The drawing under review shows one solid part. Ordinate dimensions are in mm from its lowest x, y, z. A direction names the side the tool comes from. Give positions to 0.01 mm unless a question says otherwise; leave off trailing zeros. Write each loop counter-clockwise with the first axis right and the second up, starting at its lowest first coordinate (ties: lowest second). Pieces come first, ordered by that corner, then holes. Notation, with made-up numbers: (30, -0.75) - (43, -0.75) arc R21 cw to (43, 32.25) - close; hole circle Ø9 at (32.5, 46). An arc over 180 degrees is marked (long way). Write item = value, one per line.
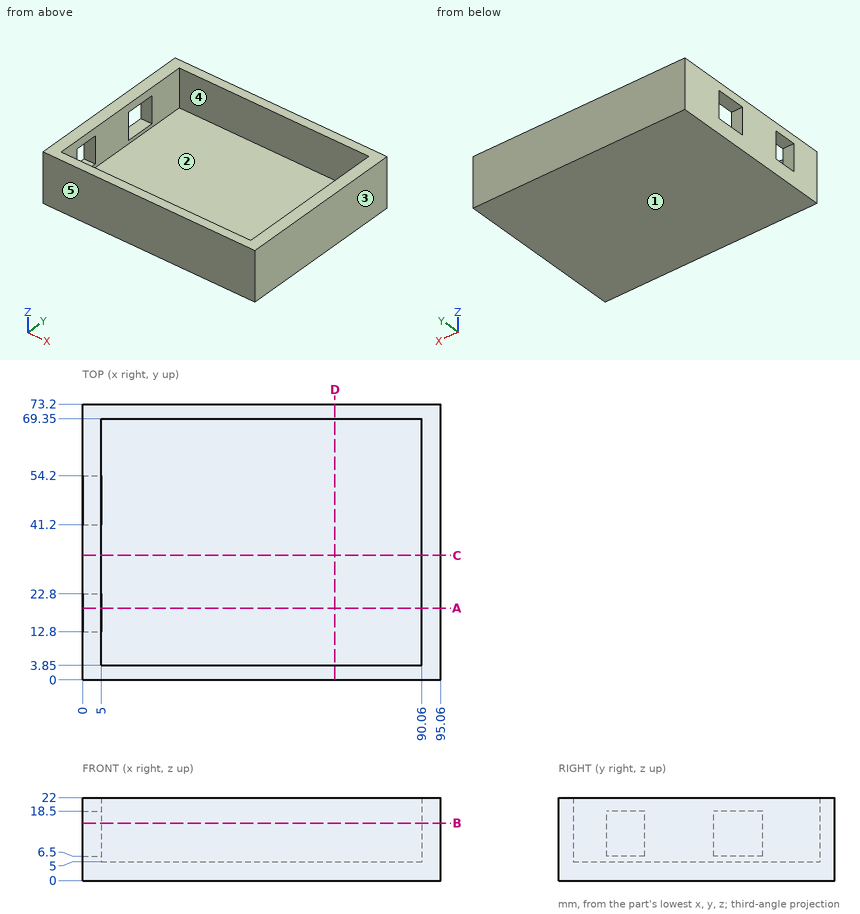
1. Take a section at B-B on z = 15.25. Give the boundary of the cut face in (x, y), and give its area (3 significant figures).
Findings below:
outline = (0, 0) - (95.06, 0) - (95.06, 73.2) - (0, 73.2) - (0, 54.2) - (5, 54.2) - (5, 69.35) - (90.06, 69.35) - (90.06, 3.85) - (5, 3.85) - (5, 12.8) - (0, 12.8) - close; (0, 22.8) - (5, 22.8) - (5, 41.2) - (0, 41.2) - close
area = 1,270 mm²
2. Insertion check: P1, Ø4, axis at x = 3, y = 48.5, coming from the -Z side; P2, Ø12, axis at x = 70, y = 35, coming from the +Z side. Each pin has a flat end and moves straight along its axis. Give the tip position at first contact, or say it passes through.
Findings below:
P1 = 0
P2 = 5
3. Take a section at D-D on x = 67. Give the boundary of the cut face in (y, z).
Findings below:
outline = (0, 0) - (73.2, 0) - (73.2, 22) - (69.35, 22) - (69.35, 5) - (3.85, 5) - (3.85, 22) - (0, 22) - close
4. Draft analysis for pull direction Y (two halves, no side actions). For the marked faces 3, 4 and 5, state which applies: +Y half, -Y half, draft (parallel to the pull), parting line (faces both ways), or undercut.
Findings below:
face_3 = draft
face_4 = undercut
face_5 = -Y half
5. Take a section at A-A on y = 19. Give the boundary of the cut face in (x, z), and give its area (3 significant figures).
Findings below:
outline = (0, 0) - (95.06, 0) - (95.06, 22) - (90.06, 22) - (90.06, 5) - (5, 5) - (5, 6.5) - (0, 6.5) - close; (0, 18.5) - (5, 18.5) - (5, 22) - (0, 22) - close
area = 585 mm²
6. Take a section at C-C on y = 33. Give the boundary of the cut face in (x, z).
Findings below:
outline = (0, 0) - (95.06, 0) - (95.06, 22) - (90.06, 22) - (90.06, 5) - (5, 5) - (5, 22) - (0, 22) - close
7. Machinability: for the marked faces 1 and 2, which of the approach directions +Z, -Z, +X, -X, +Y, -Y give a long, thin tool a straight path to every point of the face, cutting with its end or side? Answer none if there is none.
Findings below:
face_1 = -Z, +X, -X, +Y, -Y
face_2 = +Z
8. For line 1 (X direction, y = 38, z = 9); line 2 (Y direction, x = 79.5, z = 7.25); line 3 (Z direction, x = 48, y = 5.5), list the stretches that pass through material, from the lowest coordinate up. Write a range as from..to.
Findings below:
line_1 = 0..5, 90.06..95.06
line_2 = 0..3.85, 69.35..73.2
line_3 = 0..5
